```python
from build123d import *

# Parameters (mm, degrees)
SZKIC1_W                   = 120
SZKIC1_H                   = 200
ODGI_CIE_BAZOWE1_DEPTH     = 3
ODGI_CIE_DOOKOLNE1_DEPTH   = 120
ODGI_CIE_DOOKOLNE1_2_DEPTH = 120
WYTNIJ_WYCI_GNI_CIE1_REACH = 193.554
SZKIC7_R                   = 4
SZKIC7_W                   = 75.41506457
SZKIC7_H                   = 27.105706619
ZAOKR_GLENIE1_R            = 3


# Read off the part's stored shape, not the designer's step: Odgięcie dookolne1
# Sheet-metal steps are written as plain solids
with BuildPart() as part:
    # Szkic1 → Odgięcie bazowe1 (new body)
    with BuildSketch(Plane.XY):
        with Locations((60, 100)):
            Rectangle(SZKIC1_W, SZKIC1_H)
    extrude(amount=-ODGI_CIE_BAZOWE1_DEPTH)

    # Odgięcie dookolne1 outline → Odgięcie dookolne1 (cut)
    with BuildSketch(Plane.YZ):
        with BuildLine():
            Line((200, 0), (197.911617043, 0))
            ThreePointArc((197.911617043, 0), (196.615806823, -2.154295979), (194.248339822, -3))
            Line((194.248339822, -3), (200, -3))
            Line((200, -3), (200, 0))
        make_face()
    extrude(amount=ODGI_CIE_DOOKOLNE1_DEPTH, mode=Mode.SUBTRACT)

    # Odgi_cie dookolne1 2 outline → Odgi_cie dookolne1 2 (add)
    with BuildSketch(Plane.YZ):
        with BuildLine():
            Line((159.401451516, 44.178703704), (157.19251633, 42.14877628))
            Line((157.19251633, 42.14877628), (194.790707041, 1.235014847))
            ThreePointArc((194.790707041, 1.235014847), (194.922769928, 0.440418313), (194.248339822, 0))
            Line((194.248339822, 0), (197.911617043, 0))
            ThreePointArc((197.911617043, 0), (197.847182685, 1.74184107), (196.999642226, 3.264942271))
            Line((196.999642226, 3.264942271), (159.401451516, 44.178703704))
        make_face()
    extrude(amount=ODGI_CIE_DOOKOLNE1_2_DEPTH)

    # Szkic7 → Wytnij-wyciągnięcie1 (cut, up to next)
    with BuildSketch(Plane(origin=(0, 108.430992275, 99.643958017), x_dir=(1, 0, 0), z_dir=(0, 0.7363117283974429, 0.6766424747415508)), mode=Mode.PRIVATE) as wytnij_wyci_gni_cie1_sk1:
        with Locations(Location((105.046682515, 92.762095307, 0), (0, 0, 270))):
            Circle(SZKIC7_R)
    wytnij_wyci_gni_cie1_tool1 = extrude(wytnij_wyci_gni_cie1_sk1.sketch, amount=-WYTNIJ_WYCI_GNI_CIE1_REACH, mode=Mode.PRIVATE) & part.part
    # Szkic7 → Wytnij-wyciągnięcie1 (cut, up to next)
    with BuildSketch(Plane(origin=(0, 108.430992275, 99.643958017), x_dir=(1, 0, 0), z_dir=(0, 0.7363117283974429, 0.6766424747415508)), mode=Mode.PRIVATE) as wytnij_wyci_gni_cie1_sk2:
        with Locations((49.764969339, 99.719590592)):
            Rectangle(SZKIC7_W, SZKIC7_H)
    wytnij_wyci_gni_cie1_tool2 = extrude(wytnij_wyci_gni_cie1_sk2.sketch, amount=-WYTNIJ_WYCI_GNI_CIE1_REACH, mode=Mode.PRIVATE) & part.part
    add(wytnij_wyci_gni_cie1_tool1.solids().sort_by_distance((105.046683, 171.197766, 31.342139))[0], mode=Mode.SUBTRACT)
    add(wytnij_wyci_gni_cie1_tool2.solids().sort_by_distance((49.764969, 175.905503, 26.219254))[0], mode=Mode.SUBTRACT)

    # Zaokrąglenie1
    zaokr_glenie1_edges = [part.edges().sort_by_distance(p)[0] for p in [
        (0, 158.296983923, 43.163739992),
        (120, 158.296983923, 43.163739992),
        (120, 0, -1.5),
        (0, 0, -1.5),
    ]]
    fillet(zaokr_glenie1_edges, radius=ZAOKR_GLENIE1_R)


solid = part.part
```
Source: CAD feature listing. Evaluate the final solid. Frame: model axes, mm. A direction names the side the tool comes from. Coordinates: 2 decimals unless noted, no trailing zeros. Order: outer loops, then holes, each group sorted by start corner. A loop starts at its lowest first (then second) coordinate and runs counter-clockwise, first axis right, second up. Notation, with made-up numbers: (67.5, -21.75) - (124.5, -21.75) arc R15 cw to (124.5, -1.75) - close; hole circle Ø2 at (59.25, 73.25). An arc over 180 degrees is marked (long way). One line per item, written item: value.
1) Mould query, pull axis Z, two halves, no side actions, for faces 3 (the face through (107.75, 172.1, 28.17)), 4 (the face through (59.16, 184.08, 12.89)), 5 (the face through (120, 114.5, -0.4)), 6 (the face through (0.9, 158.86, 42.52)). Classes: released by +Z, released by -Z, zero draft, split by the parting line, or undercut.
Computed values:
face 3: undercut
face 4: undercut
face 5: zero draft
face 6: released by +Z
2) Cut plane B-B on y = 13.5. Output: boundary loops of the cut face in (x, z), plus the area to 3 significant figures.
Computed values:
outline: (0, -3) - (120, -3) - (120, 0) - (0, 0) - close
area: 360 mm^2
3) Ray query, line 1 (Z direction, x = 21, y = 52); line 2 (Z direction, x = 33, y = 160); line 3 (Y direction, x = 76.5, z = 35). Return the intervals inside material, ascending. Write a range as [from, to].
Computed values:
line 1: z = [-3, 0]
line 2: z = [-3, 0], [39.09, 43.53]
line 3: y = [163.76, 165.43]
4) Reachability of faces 1 (the face through (59, 98, 0)), 2 (the face through (59.16, 186.82, 14.34)) from +Z, -Z, +X, -X, +Y, -Y: full face, straight path, thin tool, end or side. Return the list, or none.
Computed values:
face 1: +X, -X, -Y
face 2: +Z, +X, -X, +Y
5) Cut plane C-C on z = 10. Output: boundary loops of the cut face in (x, y), plus the area to 3 significant figures.
Computed values:
outline: (0, 186.74) - (120, 186.74) - (120, 190.81) - (0, 190.81) - close
area: 489 mm^2
6) Cut plane A-A on x = 79.5. Output: boundary loops of the cut face in (y, z), plus the area to 3 significant figures.
Computed values:
outline: (0, -3) - (194.25, -3) arc R3.74 ccw to (197, 3.26) - (185.08, 16.24) - (182.87, 14.21) - (194.79, 1.24) arc R0.74 cw to (194.25, 0) - (0, 0) - close; (157.19, 42.15) - (164.53, 34.17) - (166.74, 36.2) - (159.4, 44.18) - close
area: 684 mm^2
7) Contact query for flat-ended pins moving along their axis: pin 1 (3 mm diameter, centred on x = 99, z = 8.5, fed in from +Y); pin 2 (8 mm diameter, centred on x = 56.5, z = 34.5, fed in from -Y). Output: stop coordinate, or through.
Computed values:
pin 1: stops at y = 193.57
pin 2: stops at y = 160.55
